```python
from build123d import *

# Parameters (mm, degrees)
F0_W     = 304.8
F0_H     = 19.05
F1_DEPTH = 31.75
F2_SIZE  = 9.52499
F3_W     = 38.1
F3_H     = 9.525
F4_DEPTH = 9.525
F5_SIZE  = 9.52499


# Not quite as in the source:
# - a fillet or chamfer is up to 0.001 mm smaller than in the source, because OpenCascade refuses the exact size
# - a pattern or mirror of a feature is missing from the dataset's text; its kind, count and spacing are read off the source's solid


with BuildPart() as f1:
    # F0 (on Top) → F1 (new body)
    with BuildSketch(Plane.XY):
        Rectangle(F0_W, F0_H)
    extrude(amount=F1_DEPTH)

    # F2 (size 9.525 in the source; OpenCascade refuses exactly that, so slightly less here)
    f2_edges = [f1.edges().sort_by_distance(p)[0] for p in [
        (0, -9.525, 31.75),
        (0, 9.525, 31.75),
    ]]
    chamfer(f2_edges, length=F2_SIZE)

    # F3 (on face) → F4 (join)
    with BuildSketch(Plane.YZ.offset(152.4)):
        with Locations((0, 4.7625)):
            Rectangle(F3_W, F3_H)
    f4 = extrude(amount=F4_DEPTH)

    # F4_copies: F4 across plane
    add(f4.mirror(Plane(origin=(0, 0, 0), x_dir=(0, 0, -1), z_dir=(-1, 0, 0))))

    # F5 (size 9.525 in the source; OpenCascade refuses exactly that, so slightly less here)
    f5_edges = [f1.edges().sort_by_distance(p)[0] for p in [
        (152.4, -9.525, 4.7625),
        (152.4, 9.525, 4.7625),
        (-152.4, -9.525, 4.7625),
        (-152.4, 9.525, 4.7625),
    ]]
    chamfer(f5_edges, length=F5_SIZE)


solid = f1.part
```
Build history of the part. All positions in model axes, mm. A direction names the side the tool comes from. Round coordinates to 2 decimals unless told otherwise and drop trailing zeros. Write each loop counter-clockwise with the first axis right and the second up, starting at its lowest first coordinate (ties: lowest second). Pieces come first, ordered by that corner, then holes. Notation, with made-up numbers: (15, 50) -> (47, 50) arc R13 cw to (47, 57) -> close; hole circle Ø11 at (80.25, -26.75). An arc over 180 degrees is marked (long way). Put each result on its own line as item: value.
Item 1: Slice it at A-A, the plane y = -4. Give the cut face in (x, z) (3 decimals), plus the area to 3 significant figures.
Here are the results:
outline: (-161.925, 0) -> (161.925, 0) -> (161.925, 9.525) -> (152.4, 9.525) -> (152.4, 27.75) -> (-152.4, 27.75) -> (-152.4, 9.525) -> (-161.925, 9.525) -> close
area: 8,640 mm^2
Item 2: Two-plate mould, pull along X, no slides. Class faces 1 (the face through (161.925, 0, 5)), 2 (the face through (157, -19.05, 5)), 3 (the face through (-161.925, 0, 5)), 4 (the face through (-2, 9.525, 11)): pulls with the +X half, pulls with the -X half, needs draft (parallel to the pull), parting line crosses it, or undercut.
Here are the results:
face 1: pulls with the +X half
face 2: needs draft
face 3: pulls with the -X half
face 4: undercut
Item 3: Tool access for faces 5 (the face through (-152.4, 0, 18)), 6 (the face through (152.4, 0, 18)), 7 (the face through (-147.57, -14.22, 4.7)), 8 (the face through (147.57, 14.22, 4.7)): list every direction of +Z, -Z, +X, -X, +Y, -Y with a clear straight run to the whole face (end or side of a thin tool).
Here are the results:
face 5: +Z, -X, +Y, -Y
face 6: +Z, +X, +Y, -Y
face 7: +Z, -Z, -Y
face 8: +Z, -Z, +Y
Item 4: Wall check: probe 1 along Y at (x, z) = (-72, 9.5) (3 decimals); probe 2 along X at (y, z) = (-2.5, 12.5); probe 3 along X at (y, z) = (17, 2) (3 decimals). Give the ranges that are in metal, low to high. Write a range as from..to.
Here are the results:
probe 1: y = -9.525..9.525
probe 2: x = -152.4..152.4
probe 3: x = -161.925..-150.35, 150.35..161.925
Item 5: Slice it at D-D, the plane y = -15.5. Give the cut face in (x, z) (3 decimals).
Here are the results:
outline: (-161.925, 0) -> (-148.85, 0) -> (-148.85, 9.525) -> (-161.925, 9.525) -> close; (148.85, 0) -> (161.925, 0) -> (161.925, 9.525) -> (148.85, 9.525) -> close
Item 6: Flat gauge pins, fed straight in: P1, Ø5.5, axis at y = -2, z = 25, coming from the -X side; P2, Ø6, axis at x = -86, z = 25.5, coming from the -Y side; P3, Ø4, axis at x = 124.5, y = 4.5, coming from the +Z side. Where does each tip first touch, or does it go through?
Here are the results:
P1: stops at x = -152.4
P2: stops at y = -9.25
P3: stops at z = 29.25
